```python
from build123d import *

# Parameters (mm, degrees)
F0_R          = 5.3435268043
F0_R_2        = 4.397766481
F1_DEPTH      = 4.9784
F2_R          = 4.6160122021
F3_DEPTH      = 1.016
F4_R          = 3.0366866858
F5_DEPTH      = 25.4
F5_DEPTH_BACK = 25.4


with BuildPart() as f1:
    # F0 (on Front) → F1 (new body)
    with BuildSketch(Plane.XZ):
        Circle(F0_R)
        Circle(F0_R_2, mode=Mode.SUBTRACT)
    extrude(amount=F1_DEPTH)

    # F2 (on Front) → F3 (join)
    with BuildSketch(Plane.XZ):
        Circle(F2_R)
    extrude(amount=F3_DEPTH)

    # F4 (on Front) → F5 (cut, two sides)
    with BuildSketch(Plane.XZ) as f5_sk:
        Circle(F4_R)
    extrude(amount=-F5_DEPTH, mode=Mode.SUBTRACT)
    extrude(f5_sk.sketch, amount=F5_DEPTH_BACK, mode=Mode.SUBTRACT)


solid = f1.part
```
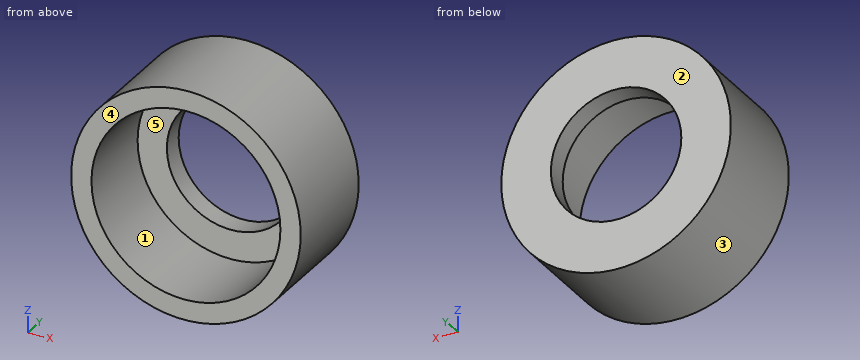
Could you check a few things on this model? Use its own coordinates, in mm. Face numbers are marked on the shaded views. A direction names the side the tool comes from. Coordinates: 2 decimals unless noted, no trailing zeros. Write each loop counter-clockwise with the first axis right and the second up, starting at its lowest first coordinate (ties: lowest second). Pieces come first, ordered by that corner, then holes. Notation, with made-up numbers: M 48,25 L 60,25 A24 cw 60,57 Z; hole C 55.25,17 d2. An arc over 180 degrees is marked long. Answer as CSV lines item,"result". Start each with the question number.
1) I want a section at A-A, the plane z = 0. Please give me the cut outline in (x, y), and give its area (3 significant figures).
2) For P1, Ø1, axis at y = -2.5, z = 1.5, coming from the -X side; P2, Ø5.5, axis at x = 0, z = 0, coming from the +Y side; P3, Ø1, axis at x = -2, y = -4.5, coming from the +Z side; P4, Ø1, axis at y = -4, z = -0.5, coming from the -X side, each with a flat end and sliding along its axis, tell me the tip position at first contact or that it passes through.
3) I want a section at B-B, the plane x = 0. Please give me the cut outline in (y, z), and give its area (3 significant figures).
4) Please list where these lines run through material, in increasing order: line 1 (Z direction, x = 0, y = -2.6); line 2 (X direction, y = -4, z = 3.75); line 3 (Z direction, x = 0, y = -0.5). Write a range as from..to.
5) I want a section at C-C, the plane y = -1.6. Please give me the cut outline in (x, z).
6) For the marked faces 1 and 2, which set-ups out of +Z, -Z, +X, -X, +Y, -Y let a thin tool reach every point of the face, with its end or its side?
7) We'd pull the mould along X, two halves only. Please class the marked faces 3, 4 and 5: +X half, -X half, draft (parallel to the pull), parting line (faces both ways), or undercut.
8) I want a section at D-D, the plane z = 3.25. Please give me the cut outline in (x, y), and give its area (3 significant figures).
Data:
1,outline,"M -5.34,-4.98 L -4.4,-4.98 L -4.4,-1.02 L -3.04,-1.02 L -3.04,0 L -5.34,0 Z; M 3.04,-1.02 L 4.4,-1.02 L 4.4,-4.98 L 5.34,-4.98 L 5.34,0 L 3.04,0 Z"
1,area,"12.2 mm^2"
2,P1,"stops at x = -5.25"
2,P2,"passes through"
2,P3,"stops at z = 5.13"
2,P4,"stops at x = -5.34"
3,outline,"M -4.98,-5.34 L 0,-5.34 L 0,-3.04 L -1.02,-3.04 L -1.02,-4.4 L -4.98,-4.4 Z; M -4.98,4.4 L -1.02,4.4 L -1.02,3.04 L 0,3.04 L 0,5.34 L -4.98,5.34 Z"
3,area,"12.2 mm^2"
4,line 1,"z = -5.34..-4.4, 4.4..5.34"
4,line 2,"x = -3.81..-2.3, 2.3..3.81"
4,line 3,"z = -5.34..-3.04, 3.04..5.34"
5,outline,"C 0,0 d10.69; hole C 0,0 d8.8"
6,face 1,"-Y"
6,face 2,"+Z, -Z, +X, -X, +Y"
7,face 3,"parting line"
7,face 4,"draft"
7,face 5,"undercut"
8,outline,"M -4.24,-4.98 L -2.96,-4.98 L -2.96,-1.02 L 2.96,-1.02 L 2.96,-4.98 L 4.24,-4.98 L 4.24,0 L -4.24,0 Z"
8,area,"18.8 mm^2"
